```python
from build123d import *

# Parameters (mm, degrees)
BOX_W             = 1
BOX_H             = 2
BOX_DEPTH         = 1
ARRAY_COUNT       = 8
CYLINDER001_R     = 2
CYLINDER001_DEPTH = 10
CYLINDER_R        = 3
CYLINDER_DEPTH    = 15


with BuildPart() as array:
    # Box → Box (new body)
    with BuildSketch(Plane(origin=(0, 1, 14), x_dir=(1, 0, 0), z_dir=(0, 0, 1))):
        with Locations((0.5, 1)):
            Rectangle(BOX_W, BOX_H)
    extrude(amount=BOX_DEPTH)

    # Array: Array ×8 about axis
    array_axis = Axis((0, 0, 0), (0, 0, 1))


with BuildPart() as array_1:
    add(array.part)
    for i in range(1, ARRAY_COUNT):
        add(array.part.rotate(array_axis, i * 360 / ARRAY_COUNT))


with BuildPart() as cilindro:
    # Cylinder001 → Cylinder001 (new body)
    with BuildSketch(Plane.XY.offset(13)):
        Circle(CYLINDER001_R)
    extrude(amount=CYLINDER001_DEPTH)


with BuildPart() as cut001:
    # Cylinder → Cylinder (new body)
    with BuildSketch(Plane.XY):
        Circle(CYLINDER_R)
    extrude(amount=CYLINDER_DEPTH)

    # Cut: cut Cilindro
    add(cilindro.part, mode=Mode.SUBTRACT)

    # Cut001: cut Array
    add(array_1.part, mode=Mode.SUBTRACT)


solid = cut001.part
```
Geometry check sheet. Reference: the model listing, model coordinates, mm. A direction names the side the tool comes from. Round coordinates to 2 decimals unless told otherwise and drop trailing zeros. Loops run counter-clockwise (first coordinate to the right, second up) from the corner with the lowest first, then second, coordinate; pieces in that order, holes last. Notation, with made-up numbers: (17, -18.5) - (42, -18.5) arc R5 cw to (42, -12.5) - close; hole circle Ø4 at (48, 27.5). An arc over 180 degrees is marked (long way). Write each question's results on one line, items separated by ' | '. Start each with the question number.
Q1. Thickness scan on line 1 (Y direction, x = 0, z = 13.7); line 2 (Z direction, x = 0.1, y = -0.2); line 3 (Z direction, x = -2.8, y = 0.1). Record the ranges inside material, lowest first. Write a range as [from, to].
Q2. Cross-section at C-C on z = 1.75. Enter the section's corners in (x, y).
Q3. Access from +Z, -Z, +X, -X, +Y, -Y to the whole of each face (thin tool, end or side, straight path). Record for faces 4 (the flat face through (-0.5, -2.4, 14)), 5 (the flat face through (-1, 2, 14)), 6 (the flat face through (2.4, -0.5, 14)).
Q4. Cross-section at B-B on y = -0.75. Enter the section's corners in (x, z), and give its area (3 significant figures).
Q5. Cross-section at A-A on x = 0.8. Enter the section's corners in (y, z).
Q6. Release check for a two-part mould opening along X. For faces 1 (the cylindrical face through (1.61, 2.53, 7.4)), 2 (the flat face through (-1, -2.3, 14.5)), 3 (the flat face through (2.1, -1.4, 15)) record: +X half, -X half, draft (parallel to the pull), parting line (faces both ways), or undercut.
Q7. Gauge pin test, flat ends, axial feed: P1, Ø0.5, axis at x = 2.5, y = -0.5, coming from the +Z side; P2, Ø1, axis at x = -1, y = 0.5, coming from the +Z side; P3, Ø1.1, axis at y = 2, z = 14.5, coming from the -X side. Record the tip position at first contact, or that the pin passes through.
Answers below:
1) line 1: y = [-3, -2], [2, 3] | line 2: z = [0, 13] | line 3: z = [0, 14]
2) outline: circle Ø6 at (0, 0)
3) face 4: +Z, -Y | face 5: +Z | face 6: +Z, +X
4) outline: (-2.9, 0) - (2.9, 0) - (2.9, 14) - (1.85, 14) - (1.85, 13) - (-1.85, 13) - (-1.85, 14) - (-2.16, 14) - (-2.16, 15) - (-2.9, 15) - close | area: 78.4 mm²
5) outline: (-2.89, 0) - (2.89, 0) - (2.89, 14) - (1.83, 14) - (1.83, 13) - (-1.83, 13) - (-1.83, 14) - (-2.21, 14) - (-2.21, 15) - (-2.89, 15) - close
6) face 1: parting line | face 2: undercut | face 3: draft
7) P1: stops at z = 14 | P2: stops at z = 13 | P3: stops at x = -2.63
